Geometry check sheet. Reference: the model listing, model coordinates, mm. A direction names the side the tool comes from. Round coordinates to 2 decimals unless told otherwise and drop trailing zeros. Write each loop counter-clockwise with the first axis right and the second up, starting at its lowest first coordinate (ties: lowest second). Pieces come first, ordered by that corner, then holes.
Item 1: Access from +Z, -Z, +X, -X, +Y, -Y to the whole of each face (thin tool, end or side, straight path). Record for faces 1 (the face through (0.11, 99.25, 4.7)), 2 (the face through (-7, -228.6, 5)), 3 (the face through (170.806, 281.25, 4.696)), 4 (the face through (56, -9, 9.525)), 5 (the face through (-7, 203.2, 5)).
Item 2: Cross-section at B-B (y = 248.5). Enter the section's corners in (x, z) (3 decimals).
Item 3: Scan lines: probe 1 along Y at (x, z) = (0, 4.25); probe 2 along X at (y, z) = (-292.1, 2.5) (3 decimals); probe 3 along Y at (x, z) = (-5.5, 7.5). Record each from-to range of solid material in increasing order.
Item 4: Cross-section at C-C (y = -89.5). Enter the section's corners in (x, z) (3 decimals), then the cut area to 3 significant figures.
Item 5: Cross-section at A-A (z = 3). State how many separate pieces and enclosed holes the cut face has, then the cut area to 3 significant figures.
Item 6: Draft check along Y on faces 6 (the face through (88, 284.872, 5)), 7 (the face through (0.11, -40.45, 4.7)), 8 (the face through (15.875, 247, 5)), 9 (the face through (90, -311.15, 5)). Enter one of: pulls with the +Y half, pulls with the -Y half, needs draft (parallel to the pull), parting line crosses it, or undercut.
Item 7: Depth check by flat-ended pin: P1, Ø3, axis at y = -258, z = 3, coming from the -X side (3 decimals); P2, Ø1, axis at x = -6.5, z = 9, coming from the -Y side. Enter the tip coordinate at first touch or a pass-through.
from build123d import *

# Parameters (mm, degrees)
BOSS_EXTRUDE1_DEPTH            = 9.525
V_0_377_DIAMETER_SLOT2_DEPTH   = 9.525
CUT_EXTRUDE1_REACH             = 358.93
SKETCH6_W                      = 152.4
SKETCH6_H                      = 622.3
FILLET1_R                      = 12.7
SKETCH7_R                      = 8.382
CUT_EXTRUDE2_DEPTH             = 357.929879318
SKETCH12_W                     = 38.1
SKETCH12_H                     = 107.95
SKETCH12_H_2                   = 82.55
CUT_EXTRUDE3_DEPTH             = 357.929879318
FILLET2_R                      = 6.35
F_5_16_0_3125_DIAMETER_HOLE1_D = 7.9375
SKETCH16_W                     = 158.75
SKETCH16_H                     = 26.277954941
CUT_EXTRUDE4_DEPTH             = 357.929879318
F_5_16_0_3125_DIAMETER_HOLE2_D = 7.9375
FILLET3_R                      = 12.7
CUT_EXTRUDE5_DEPTH             = 1.27


# Read off the part's stored shape, not the designer's step: V (0.377) Diameter Slot2
with BuildPart() as part:
    # Sketch1 → Boss-Extrude1 (new body)
    with BuildSketch(Plane.XY):
        with BuildLine():
            Line((-174.625, 151.522045059), (-174.625, 311.15))
            Line((-174.625, 311.15), (174.625, 311.15))
            Line((174.625, 311.15), (174.625, 151.522045059))
            ThreePointArc((174.625, 151.522045059), (66.675, -31.75), (174.625, -215.022045059))
            Line((174.625, -215.022045059), (174.625, -311.15))
            Line((174.625, -311.15), (-174.625, -311.15))
            Line((-174.625, -311.15), (-174.625, -215.022045059))
            ThreePointArc((-174.625, -215.022045059), (-66.675, -31.75), (-174.625, 151.522045059))
        make_face()
    extrude(amount=BOSS_EXTRUDE1_DEPTH)

    # V (0.377) Diameter Slot2 outline → V (0.377) Diameter Slot2 (cut)
    with BuildSketch(Plane.XY):
        with BuildLine():
            Line((4.7879, -57.8866), (4.7879, -45.2374))
            ThreePointArc((4.7879, -45.2374), (0, -40.4495), (-4.7879, -45.2374))
            Line((-4.7879, -45.2374), (-4.7879, -57.8866))
            ThreePointArc((-4.7879, -57.8866), (0, -62.6745), (4.7879, -57.8866))
        make_face()
        with BuildLine():
            ThreePointArc((4.7879, 94.4626), (0, 99.2505), (-4.7879, 94.4626))
            Line((-4.7879, 94.4626), (-4.7879, 81.8134))
            ThreePointArc((-4.7879, 81.8134), (0, 77.0255), (4.7879, 81.8134))
            Line((4.7879, 81.8134), (4.7879, 94.4626))
        make_face()
        with BuildLine():
            ThreePointArc((4.7879, -184.9374), (0, -180.1495), (-4.7879, -184.9374))
            Line((-4.7879, -184.9374), (-4.7879, -197.5866))
            ThreePointArc((-4.7879, -197.5866), (0, -202.3745), (4.7879, -197.5866))
            Line((4.7879, -197.5866), (4.7879, -184.9374))
        make_face()
    extrude(amount=V_0_377_DIAMETER_SLOT2_DEPTH, mode=Mode.SUBTRACT)

    # Sketch6 → Cut-Extrude1 (cut, up to next)
    with BuildSketch(Plane.XY.offset(9.525), mode=Mode.PRIVATE) as cut_extrude1_sk1:
        with Locations((-98.425, 0)):
            Rectangle(SKETCH6_W, SKETCH6_H)
    cut_extrude1_tool1 = extrude(cut_extrude1_sk1.sketch, amount=-CUT_EXTRUDE1_REACH, mode=Mode.PRIVATE) & part.part
    add(cut_extrude1_tool1.solids().sort_by_distance((-98.425, 0, 9.525))[0], mode=Mode.SUBTRACT)

    # Fillet1
    fillet1_edges = [part.edges().sort_by_distance(p)[0] for p in [
        (174.625, -311.15, 4.7625),
    ]]
    fillet(fillet1_edges, radius=FILLET1_R)

    # Sketch7 → Cut-Extrude2 (cut, through all)
    with BuildSketch(Plane.XY.offset(9.525)):
        with Locations((0, -197.5866)):
            Circle(SKETCH7_R)
        with Locations((0, 81.8134)):
            Circle(SKETCH7_R)
        with Locations((0, -57.8866)):
            Circle(SKETCH7_R)
    extrude(amount=-CUT_EXTRUDE2_DEPTH, mode=Mode.SUBTRACT)

    # Sketch12 → Cut-Extrude3 (cut, through all)
    with BuildSketch(Plane.XY.offset(9.525)):
        with Locations((-3.175, 257.175)):
            Rectangle(SKETCH12_W, SKETCH12_H)
        with Locations((-3.175, -269.875)):
            Rectangle(SKETCH12_W, SKETCH12_H_2)
    extrude(amount=-CUT_EXTRUDE3_DEPTH, mode=Mode.SUBTRACT)

    # Fillet2
    fillet2_edges = [part.edges().sort_by_distance(p)[0] for p in [
        (15.875, 203.2, 4.7625),
        (15.875, -228.6, 4.7625),
    ]]
    fillet(fillet2_edges, radius=FILLET2_R)

    # 5/16 (0.3125) Diameter Hole1 (through all)
    with Locations(Plane.XY.offset(9.525)):
        with Locations((85.7885, 170.688), (85.7885, 265.938)):
            Hole(F_5_16_0_3125_DIAMETER_HOLE1_D / 2)

    # Sketch16 → Cut-Extrude4 (cut, through all)
    with BuildSketch(Plane.XY.offset(9.525)):
        with Locations((95.25, 298.011022529)):
            Rectangle(SKETCH16_W, SKETCH16_H)
    extrude(amount=-CUT_EXTRUDE4_DEPTH, mode=Mode.SUBTRACT)

    # 5/16 (0.3125) Diameter Hole2 (through all)
    with Locations(Plane.XY.offset(9.525)):
        with Locations((85.7885, -234.95), (85.7885, -292.1)):
            Hole(F_5_16_0_3125_DIAMETER_HOLE2_D / 2)

    # Fillet3
    fillet3_edges = [part.edges().sort_by_distance(p)[0] for p in [
        (174.625, 284.872045059, 4.7625),
    ]]
    fillet(fillet3_edges, radius=FILLET3_R)

    # Sketch22 → Cut-Extrude5 (cut)
    with BuildSketch(Plane(origin=(0, 0, 9.525), x_dir=(-1, 0, 0), z_dir=(0, 0, -1))):
        Polygon((9.687820513, 190.5), (8.548076923, 190.5), (8.548076923, 179.102564103), (3.663461538, 179.102564103), (3.663461538, 177.8), (9.687820513, 177.8), align=None)
    extrude(amount=CUT_EXTRUDE5_DEPTH, mode=Mode.SUBTRACT)


solid = part.part
Resolved:
1. face 1: +Z, -Z
1. face 2: +Z, -Z, -X, -Y
1. face 3: +Z, -Z, +X, +Y
1. face 4: +Z, +X, -X, +Y, -Y
1. face 5: +Z, -Z, -X, +Y
2. outline: (15.875, 0) - (174.625, 0) - (174.625, 9.525) - (15.875, 9.525) - close
3. probe 1: y = -228.6 to -205.97, -180.15 to -66.27, -40.45 to 73.43, 99.25 to 203.2
3. probe 2: x = 15.875 to 81.82, 89.757 to 174.625
3. probe 3: y = -228.6 to -203.91, -191.26 to -64.21, -51.56 to 75.49, 88.14 to 203.2
4. outline: (-22.225, 0) - (74.79, 0) - (74.79, 9.525) - (-22.225, 9.525) - close
4. area: 924 mm2
5. separate pieces: 1
5. enclosed holes: 7
5. area: 81,800 mm2
6. face 6: pulls with the +Y half
6. face 7: undercut
6. face 8: needs draft
6. face 9: pulls with the -Y half
7. P1: stops at x = 15.875
7. P2: stops at y = -228.6
